```python
from build123d import *

# Parameters (mm, degrees)
F0_W     = 381
F0_H     = 381
F1_DEPTH = 317.5
F2_SIZE  = 254
F3_R     = 25.4


with BuildPart() as f1:
    # F0 (on Top) → F1 (new body)
    with BuildSketch(Plane.XY):
        Rectangle(F0_W, F0_H)
    extrude(amount=F1_DEPTH)

    # F2
    f2_edges = [f1.edges().sort_by_distance(p)[0] for p in [
        (0, -190.5, 317.5),
    ]]
    chamfer(f2_edges, length=F2_SIZE)

    # F3
    f3_edges = [f1.edges().sort_by_distance(p)[0] for p in [
        (190.5, 190.5, 158.75),
        (-190.5, 190.5, 158.75),
        (0, 190.5, 0),
        (0, 190.5, 317.5),
        (-190.5, -190.5, 31.75),
        (-190.5, -63.5, 190.5),
        (-190.5, 0, 0),
        (-190.5, 127, 317.5),
        (190.5, 127, 317.5),
        (0, 63.5, 317.5),
        (190.5, -190.5, 31.75),
        (190.5, -63.5, 190.5),
        (190.5, 0, 0),
        (0, -190.5, 0),
        (0, -190.5, 63.5),
    ]]
    fillet(f3_edges, radius=F3_R)


solid = f1.part
```
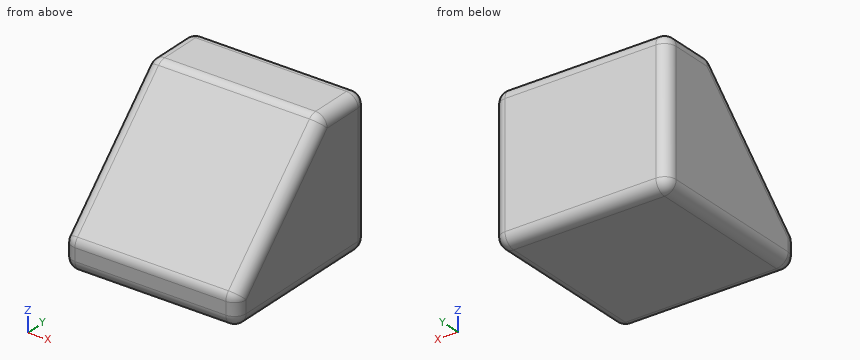
Geometry check sheet. Reference: the model listing, model coordinates, mm. Give positions to 0.01 mm unless a question says otherwise; leave off trailing zeros. Loops run counter-clockwise (first coordinate to the right, second up) from the corner with the lowest first, then second, coordinate; pieces in that order, holes last. Notation, with made-up numbers: M 69,7 L 103,7 A35 ccw 103,41 Z; hole C 36,64.25 d7. An arc over 180 degrees is marked long. Write item = value, one per line. Start each with the question number.
1. Thickness scan on probe 1 along X at (y, z) = (166, 228.5); probe 2 along Y at (x, z) = (170, 228.5); probe 3 along Y at (x, z) = (-108, 202.5). Record the ranges inside material, lowest first.
2. Section check A-A, the plane x = 80. Enter the section's corners in (y, z), plus the area to 3 significant figures.
3. Go/stop test with flat-tipped pins: P1, Ø2, axis at x = 58, z = 190.5, coming from the -Y side; P2, Ø10, axis at x = 16.5, y = -19, coming from the +Z side; P3, Ø3, axis at x = -94.5, z = 257, coming from the -Y side. Record where each tip stops, or that it passes through.
Values follow:
q1.probe_1 = -190.48 to 190.48
q1.probe_2 = -24.83 to 190.02
q1.probe_3 = -51.5 to 190.5
q2.outline = M -190.5,25.4 A25.4 ccw -165.1,0 L 165.1,0 A25.4 ccw 190.5,25.4 L 190.5,292.1 A25.4 ccw 165.1,317.5 L 74.02,317.5 A25.4 ccw 56.06,310.06 L -183.06,70.94 A25.4 ccw -190.5,52.98 Z
q2.area = 88,300 mm^2
q3.P1 = -64.5
q3.P2 = 240
q3.P3 = 1.5
